Could you check a few things on this drawing? It's one solid part, dimensions in mm from its lowest x, y, z. Round coordinates to 2 decimals unless told otherwise and drop trailing zeros. Write each loop counter-clockwise with the first axis right and the second up, starting at its lowest first coordinate (ties: lowest second). Pieces come first, ordered by that corner, then holes. Notation, with made-up numbers: (4, -12.5) -> (63, -12.5) arc R19 ccw to (63, -3.5) -> close; hole circle Ø3 at (53, 30.25). An arc over 180 degrees is marked (long way). Answer in a Markdown table with one row per item.
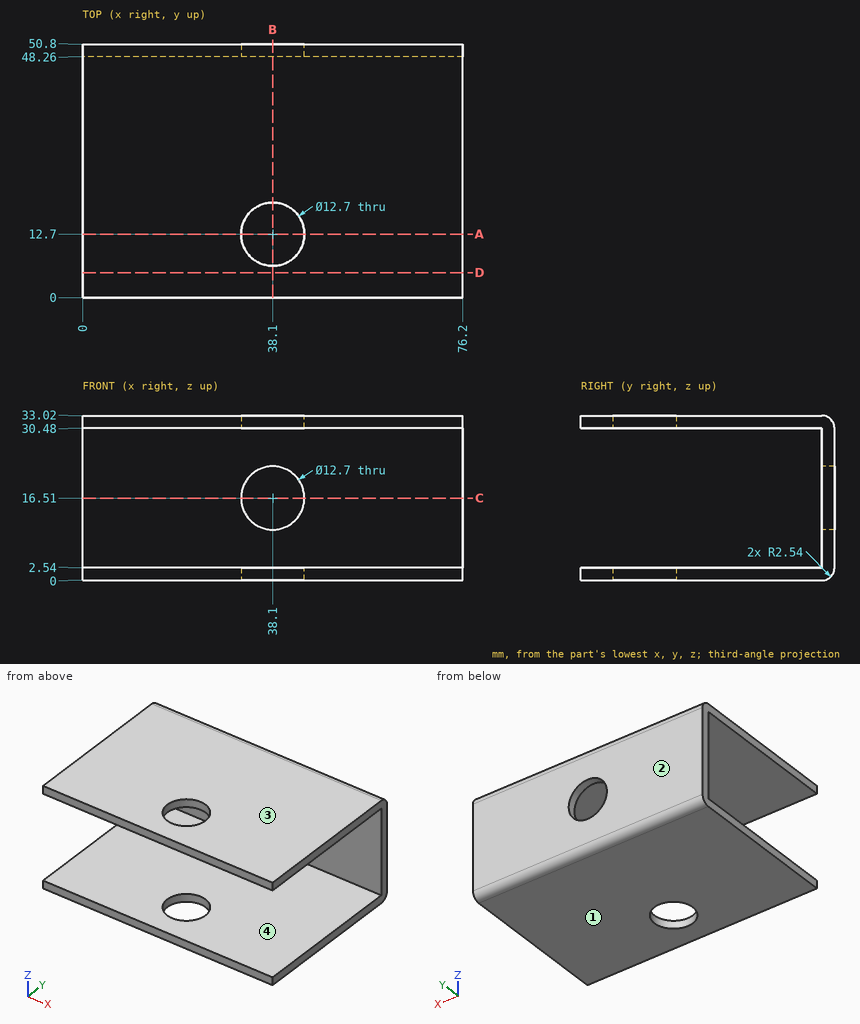
1) For pin 1 (6 mm diameter, centred on x = 21, z = 15, fed in from -Y), with a flat end and sliding along its axis, tell me the tip position at first contact or that it passes through.
Findings:
| item | result |
|---|---|
| pin 1 | stops at y = 48.26 |
2) Imagine slicing it at D-D, the plane y = 5. Please give me the cut outline in (x, z).
Findings:
| item | result |
|---|---|
| outline | (0, 0) -> (76.2, 0) -> (76.2, 2.54) -> (0, 2.54) -> close; (0, 30.48) -> (76.2, 30.48) -> (76.2, 33.02) -> (0, 33.02) -> close |
3) Thinking about a two-plate mould opening in Z: for the marked faces 1, 2, 3 and 4, which applies, +Z half, -Z half, draft (parallel to the pull), parting line (faces both ways), or undercut?
Findings:
| item | result |
|---|---|
| face 1 | -Z half |
| face 2 | draft |
| face 3 | +Z half |
| face 4 | undercut |
4) Imagine slicing it at A-A, the plane y = 12.7. Please give me the cut outline in (x, z).
Findings:
| item | result |
|---|---|
| outline | (0, 0) -> (31.75, 0) -> (31.75, 2.54) -> (0, 2.54) -> close; (0, 30.48) -> (31.75, 30.48) -> (31.75, 33.02) -> (0, 33.02) -> close; (44.45, 0) -> (76.2, 0) -> (76.2, 2.54) -> (44.45, 2.54) -> close; (44.45, 30.48) -> (76.2, 30.48) -> (76.2, 33.02) -> (44.45, 33.02) -> close |
5) Imagine slicing it at C-C, the plane z = 16.51. Please give me the cut outline in (x, y).
Findings:
| item | result |
|---|---|
| outline | (0, 48.26) -> (31.75, 48.26) -> (31.75, 50.8) -> (0, 50.8) -> close; (44.45, 48.26) -> (76.2, 48.26) -> (76.2, 50.8) -> (44.45, 50.8) -> close |
6) Imagine slicing it at B-B, the plane x = 38.1. Please give me the cut outline in (y, z), plus the area to 3 significant figures.
Findings:
| item | result |
|---|---|
| outline | (0, 0) -> (6.35, 0) -> (6.35, 2.54) -> (0, 2.54) -> close; (0, 30.48) -> (6.35, 30.48) -> (6.35, 33.02) -> (0, 33.02) -> close; (19.05, 0) -> (48.26, 0) arc R2.54 ccw to (50.8, 2.54) -> (50.8, 10.16) -> (48.26, 10.16) -> (48.26, 2.54) -> (19.05, 2.54) -> close; (19.05, 30.48) -> (48.26, 30.48) -> (48.26, 22.86) -> (50.8, 22.86) -> (50.8, 30.48) arc R2.54 ccw to (48.26, 33.02) -> (19.05, 33.02) -> close |
| area | 229 mm^2 |
7) Please list where these lines run through material, in increasing order: line 1 (Z direction, x = 63, y = 11.5); line 2 (X direction, y = 12.7, z = 0.95); line 3 (Y direction, x = 21.5, z = 8).
Findings:
| item | result |
|---|---|
| line 1 | z = 0 to 2.54, 30.48 to 33.02 |
| line 2 | x = 0 to 31.75, 44.45 to 76.2 |
| line 3 | y = 48.26 to 50.8 |
